CAD build for the part. Positions are in the model's coordinates, mm. Face numbers are marked on the shaded views. A direction names the side the tool comes from. Give positions to 0.01 mm unless a question says otherwise; leave off trailing zeros. Write each loop counter-clockwise with the first axis right and the second up, starting at its lowest first coordinate (ties: lowest second). Pieces come first, ordered by that corner, then holes. Notation, with made-up numbers: (-9, 21) -> (22, 21) arc R15 ccw to (22, 26) -> close; hole circle Ø3 at (63, 14.5). An arc over 180 degrees is marked (long way). Answer as a JSON object with one key per item and string values.
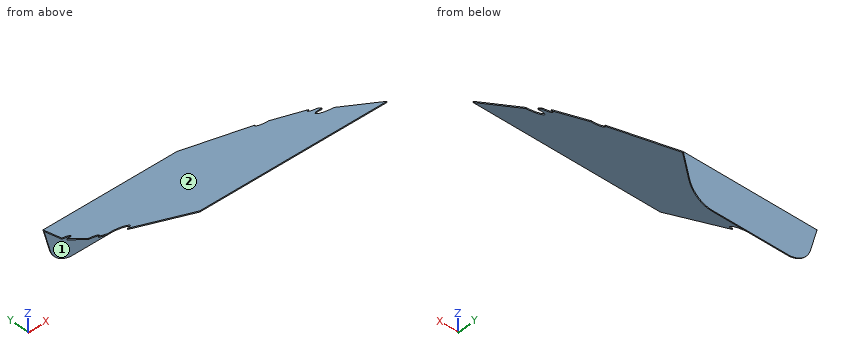
```python
from build123d import *

# Parameters (mm, degrees)
BOSS_EXTRUDE1_DEPTH = 2.54
SKETCH3_W           = 635
SKETCH3_H           = 1270
BOSS_EXTRUDE2_DEPTH = 2.54
CUT_EXTRUDE1_START  = -2.001547314
CUT_EXTRUDE1_DEPTH  = 783.891620978


# Read off the part's stored shape, not the designer's step: Cut-Extrude1
with BuildPart() as part:
    # Sketch2 → Boss-Extrude1 (new body)
    with BuildSketch(Plane(origin=(0, 0, 0), x_dir=(1, 0, 0), z_dir=(0, 1, 0))):
        with BuildLine():
            Line((-190.5, 0), (190.5, 0))
            Line((190.5, 0), (172.589792707, 64.649970609))
            ThreePointArc((172.589792707, 64.649970609), (148.320865378, 100.476994518), (107.315, 114.3))
            Line((107.315, 114.3), (-107.315, 114.3))
            ThreePointArc((-107.315, 114.3), (-148.320865378, 100.476994518), (-172.589792707, 64.649970609))
            Line((-172.589792707, 64.649970609), (-190.5, 0))
        make_face()
    extrude(amount=-BOSS_EXTRUDE1_DEPTH)

    # Sketch3 → Boss-Extrude2 (add)
    with BuildSketch(Plane(origin=(0, 0, 0), x_dir=(1, 0, 0), z_dir=(0, 0.6156614753256567, 0.7880107536067232))):
        with Locations((0, -635)):
            Rectangle(SKETCH3_W, SKETCH3_H)
    extrude(amount=-BOSS_EXTRUDE2_DEPTH)

    # Cut-Extrude1 outline → Cut-Extrude1 (cut)
    with BuildSketch(Plane.XY.offset(CUT_EXTRUDE1_START)):
        with BuildLine():
            Line((-275.07291121, -151.325406705), (-190.5, 0))
            Line((-190.5, 0), (-571.5, 0))
            Line((-571.5, 0), (-571.5, -1524))
            Line((-571.5, -1524), (571.5, -1524))
            Line((571.5, -1524), (571.5, 0))
            Line((571.5, 0), (190.5, 0))
            Line((190.5, 0), (275.07291121, -151.325406705))
            ThreePointArc((275.07291121, -151.325406705), (268.12028899, -171.183230141), (286.984028398, -180.501569203))
            Line((286.984028398, -180.501569203), (312.982021819, -276.089162217))
            ThreePointArc((312.982021819, -276.089162217), (301.277723529, -291.035795076), (312.269080611, -306.514247899))
            Line((312.269080611, -306.514247899), (305.43807978, -327.663433526))
            ThreePointArc((305.43807978, -327.663433526), (272.877245274, -346.141774353), (294.096224924, -376.98674033))
            Line((294.096224924, -376.98674033), (266.7, -571.921009662))
            Line((266.7, -571.921009662), (-266.7, -571.921009662))
            Line((-266.7, -571.921009662), (-294.096224924, -376.98674033))
            ThreePointArc((-294.096224924, -376.98674033), (-272.877245274, -346.141774353), (-305.43807978, -327.663433526))
            Line((-305.43807978, -327.663433526), (-312.269080611, -306.514247899))
            ThreePointArc((-312.269080611, -306.514247899), (-301.277723529, -291.035795076), (-312.982021819, -276.089162217))
            Line((-312.982021819, -276.089162217), (-286.984028398, -180.501569203))
            ThreePointArc((-286.984028398, -180.501569203), (-268.12028899, -171.183230141), (-275.07291121, -151.325406705))
        make_face()
        with BuildLine():
            Line((-317.5, -275.536581572), (-317.5, -307.278791903))
            ThreePointArc((-317.5, -307.278791903), (-333.023366919, -291.407686738), (-317.5, -275.536581572))
        make_face(mode=Mode.SUBTRACT)
        with BuildLine():
            ThreePointArc((-317.5, -367.657699848), (-323.031221688, -351.833931384), (-317.5, -336.01016292))
            Line((-317.5, -336.01016292), (-317.5, -367.657699848))
        make_face(mode=Mode.SUBTRACT)
        with BuildLine():
            Line((317.5, -367.657699848), (317.5, -336.01016292))
            ThreePointArc((317.5, -336.01016292), (323.031221688, -351.833931384), (317.5, -367.657699848))
        make_face(mode=Mode.SUBTRACT)
        with BuildLine():
            Line((317.5, -307.278791903), (317.5, -275.536581572))
            ThreePointArc((317.5, -275.536581572), (333.023366919, -291.407686738), (317.5, -307.278791903))
        make_face(mode=Mode.SUBTRACT)
    extrude(amount=CUT_EXTRUDE1_DEPTH, mode=Mode.SUBTRACT)


solid = part.part
```
1) Wall check: probe 1 along Y at (x, z) = (34, 131.5); probe 2 along Y at (x, z) = (-84, 129); probe 3 along Z at (x, y) = (49, -90). Give the ranges that are in metal, low to high.
Model answer:
{"probe 1": "y = -172.44 to -168.31", "probe 2": "y = -169.24 to -165.11", "probe 3": "z = 67.09 to 70.32"}
2) Pin check, flat tips, straight feed: pin 1 (3 mm diameter, centred on x = -225.5, y = -399.5, fed in from +Z); pin 2 (2 mm diameter, centred on x = 165.5, z = 130.5, fed in from +Y); pin 3 (1 mm diameter, centred on x = 119.5, y = -512, fed in from -Z). Stop position of each tip, or through.
Model answer:
{"pin 1": "stops at z = 313.3", "pin 2": "stops at y = -165.75", "pin 3": "stops at z = 396.4"}
3) Slice it at B-B (y = -39.5). List the corners of the cut face in (x, z), then the cut area to 3 significant figures.
Model answer:
{"outline": "(-212.58, 27.64) -> (212.58, 27.64) -> (212.58, 30.86) -> (-212.58, 30.86) -> close", "area": "1,370 mm2"}
4) 3-axis set-ups, long thin cutter, end or side, ignore diameter. For the marked faces 1 and 2: which of +Z, -Z, +X, -X, +Y, -Y reach the whole face in a straight line?
Model answer:
{"face 1": "-Z, +X, -X, -Y", "face 2": "+Z, +X, -X, +Y"}
5) Slice it at A-A (x = -89.5). List the corners of the cut face in (y, z).
Model answer:
{"outline": "(-571.92, 443.61) -> (-2.54, -1.24) -> (-2.54, -114.3) -> (0, -114.3) -> (0, 0) -> (-571.92, 446.83) -> close"}
6) Slice it at C-C (z = 76). List the corners of the cut face in (x, y), then the cut area to 3 significant figures.
Model answer:
{"outline": "(-247.17, -101.4) -> (247.17, -101.4) -> (244.87, -97.28) -> (-244.87, -97.28) -> close", "area": "2,030 mm2"}
